```python
from build123d import *

# Parameters (mm, degrees)
SKETCH2_R               = 10
BOSS_EXTRUDE1_DEPTH     = 30
CUT_EXTRUDE1_START      = -10
SKETCH3_R               = 10
SKETCH3_R_2             = 7.5
CUT_EXTRUDE1_DEPTH      = 10
CUT_EXTRUDE3_DEPTH      = 10
CUT_EXTRUDE3_DEPTH_BACK = 10
SKETCH5_R               = 2
FILLET2_R               = 10
BOSS_EXTRUDE2_START     = -67.5
SKETCH7_R               = 10
BOSS_EXTRUDE2_DEPTH     = 67.5
SKETCH8_R               = 50
SKETCH8_R_2             = 10
CUT_EXTRUDE6_DEPTH      = 107.770782567
SKETCH10_R              = 10.75
SKETCH10_R_2            = 10
BOSS_EXTRUDE3_DEPTH     = 15
SKETCH11_R              = 12.5
BOSS_EXTRUDE4_DEPTH     = 3


with BuildPart() as part:
    # Sketch1 → Revolve1 (revolve)
    with BuildSketch(Plane.XY):
        Polygon((50, 25), (0, 25), (0, 22.5), (45, 22.5), (45, -22.5), (0, -22.5), (0, -25), (50, -25), align=None)
    revolve(axis=Axis((0, -25, 0), (0, 1, 0)))

    # Sketch2 → Boss-Extrude1 (add)
    with BuildSketch(Plane(origin=(0, 25, 0), x_dir=(1, 0, 0), z_dir=(0, 1, 0))):
        with Locations(Location((0, 0, 0), (0, 0, 180))):
            Circle(SKETCH2_R)
    extrude(amount=BOSS_EXTRUDE1_DEPTH)

    # Sketch3 → Cut-Extrude1 (cut)
    with BuildSketch(Plane(origin=(0, 55, 0), x_dir=(1, 0, 0), z_dir=(0, 1, 0)).offset(CUT_EXTRUDE1_START)):
        with Locations(Location((0, 0, 0), (0, 0, 180))):
            Circle(SKETCH3_R)
        with Locations(Location((0, 0, 0), (0, 0, 180))):
            Circle(SKETCH3_R_2, mode=Mode.SUBTRACT)
    extrude(amount=CUT_EXTRUDE1_DEPTH, mode=Mode.SUBTRACT)

    # Sketch5 → Cut-Extrude3 (cut, two sides: drawn at the far end of the back side and taken through both)
    with BuildSketch(Plane(origin=(0, 0, 0), x_dir=(0, 0, -1), z_dir=(1, 0, 0)).offset(-CUT_EXTRUDE3_DEPTH_BACK)):
        with Locations(Location((0, 50, 0), (0, 0, 180))):
            Circle(SKETCH5_R)
    extrude(amount=CUT_EXTRUDE3_DEPTH + CUT_EXTRUDE3_DEPTH_BACK, mode=Mode.SUBTRACT)

    # Fillet2
    fillet2_edges = [part.edges().sort_by_distance(p)[0] for p in [
        (-50, 25, 0),
    ]]
    fillet(fillet2_edges, radius=FILLET2_R)

    # Sketch7 → Boss-Extrude2 (add)
    with BuildSketch(Plane(origin=(0, 45, 0), x_dir=(1, 0, 0), z_dir=(0, 1, 0)).offset(BOSS_EXTRUDE2_START)):
        with Locations(Location((0, 0, 0), (0, 0, 180))):
            Circle(SKETCH7_R)
    extrude(amount=BOSS_EXTRUDE2_DEPTH)

    # Sketch8 → Cut-Extrude6 (cut, through all)
    with BuildSketch(Plane(origin=(0, 55, 0), x_dir=(1, 0, 0), z_dir=(0, 1, 0))):
        Circle(SKETCH8_R)
        with Locations(Location((0, 0, 0), (0, 0, 180))):
            Circle(SKETCH8_R_2, mode=Mode.SUBTRACT)
    extrude(amount=-CUT_EXTRUDE6_DEPTH, mode=Mode.SUBTRACT)

    # Sketch10 → Boss-Extrude3 (add)
    with BuildSketch(Plane.XZ.offset(25)):
        Circle(SKETCH10_R)
        Circle(SKETCH10_R_2, mode=Mode.SUBTRACT)
    extrude(amount=-BOSS_EXTRUDE3_DEPTH)

    # Sketch11 → Boss-Extrude4 (add)
    with BuildSketch(Plane(origin=(0, -10, 0), x_dir=(1, 0, 0), z_dir=(0, 1, 0))):
        with Locations(Location((0, 0, 0), (0, 0, 180))):
            Circle(SKETCH11_R)
    extrude(amount=BOSS_EXTRUDE4_DEPTH)


solid = part.part
```
CAD build for the part. Positions are in the model's coordinates, mm. A direction names the side the tool comes from. Give positions to 0.01 mm unless a question says otherwise; leave off trailing zeros. Loops run counter-clockwise (first coordinate to the right, second up) from the corner with the lowest first, then second, coordinate; pieces in that order, holes last. Notation, with made-up numbers: (76, -34) - (82, -34) arc R10 cw to (82, -20) - close; hole circle Ø7 at (-14, 68.25). An arc over 180 degrees is marked (long way). Put each result on its own line as item: value.
Q1. Slice it at C-C (y = -8). Give the cut face in (x, z).
Filled in:
outline: circle Ø25 at (0, 0)
Q2. Mould opens along Y. For faces 4 (the face through (0, 55, 0)), 5 (the face through (-0.105, 51.774, 0.923)), 6 (the face through (-1.4, -17.6, 10.66)) say: pulls with the +Y half, pulls with the -Y half, needs draft (parallel to the pull), parting line crosses it, or undercut.
Filled in:
face 4: pulls with the +Y half
face 5: undercut
face 6: needs draft
Q3. Slice it at B-B (x = 0). Give the cut face in (y, z).
Filled in:
outline: (-25, -10.75) - (-10, -10.75) - (-10, -12.5) - (-7, -12.5) - (-7, -10) - (45, -10) - (45, -7.5) - (55, -7.5) - (55, 7.5) - (45, 7.5) - (45, 10) - (-7, 10) - (-7, 12.5) - (-10, 12.5) - (-10, 10.75) - (-25, 10.75) - close; hole circle Ø4 at (50, 0)
Q4. Slice it at A-A (z = 0). Give the cut face in (x, y), plus the area to 3 significant figures.
Filled in:
outline: (-12.5, -10) - (-10.75, -10) - (-10.75, -25) - (10.75, -25) - (10.75, -10) - (12.5, -10) - (12.5, -7) - (10, -7) - (10, 45) - (7.5, 45) - (7.5, 48) - (-7.5, 48) - (-7.5, 45) - (-10, 45) - (-10, -7) - (-12.5, -7) - close; (-7.5, 52) - (7.5, 52) - (7.5, 55) - (-7.5, 55) - close
area: 1,530 mm²
Q5. Flat gauge pins, fed straight in: pin 1 (1.5 mm diameter, centred on x = 10, y = 24.5, fed in from -Z); pin 2 (1.5 mm diameter, centred on x = -5.5, y = 40.5, fed in from -Z); pin 3 (12 mm diameter, centred on y = 20, z = 2.5, fed in from +X). Where does each tip first touch, or does it go through?
Filled in:
pin 1: stops at z = -3.8
pin 2: stops at z = -8.8
pin 3: stops at x = 10
Q6. Tool access for faces 1 (the face through (10, 19, 0)), 2 (the face through (3.76, -10, 10.24)), 3 (the face through (-11.923, -8.521, 3.755)): list every direction of +Z, -Z, +X, -X, +Y, -Y with a clear straight run to the whole face (end or side of a thin tool).
Filled in:
face 1: +Y
face 2: -Y
face 3: +Y, -Y
Q7. Probe line 1 along Y through (x, z) = (0, 0); line 2 along Y through (x, z) = (-9.5, -1.5); line 3 along Z through (x, y) = (-0.25, 50). List the from-to ranges inside material, lowest first.
Filled in:
line 1: y = -25 to 48, 52 to 55
line 2: y = -25 to 45
line 3: z = -7.5 to -2, 2 to 7.5
Q8. Slice it at D-D (z = -6.75). Give the cut face in (x, y), plus the area to 3 significant figures.
Filled in:
outline: (-10.52, -10) - (-8.37, -10) - (-8.37, -25) - (8.37, -25) - (8.37, -10) - (10.52, -10) - (10.52, -7) - (7.38, -7) - (7.38, 45) - (3.27, 45) - (3.27, 55) - (-3.27, 55) - (-3.27, 45) - (-7.38, 45) - (-7.38, -7) - (-10.52, -7) - close
area: 1,150 mm²
